Check sheet for the modelled part. Datum: model origin and axes. Units: mm. A direction names the side the tool comes from. Coordinates: 2 decimals unless noted, no trailing zeros. Loops run counter-clockwise (first coordinate to the right, second up) from the corner with the lowest first, then second, coordinate; pieces in that order, holes last.
```python
from build123d import *

# Parameters (mm, degrees)
SKETCH2_R          = 1.5
CUT_EXTRUDE1_DEPTH = 4
SKETCH3_R          = 8.057142585
CUT_EXTRUDE2_DEPTH = 1


with BuildPart() as part:
    # Sketch1 → Revolve2 (revolve)
    with BuildSketch(Plane(origin=(0, 0, 0), x_dir=(0, 0, -1), z_dir=(1, 0, 0))):
        with BuildLine():
            Line((0, 0), (0, 15.5))
            Line((0, 15.5), (2, 15.5))
            Line((2, 15.5), (2, 17.5))
            Line((2, 17.5), (0, 17.5))
            Line((0, 17.5), (0, 20))
            add(Edge.make_bspline(
                [(0, 20), (1.556141404, 22.961218059), (4.442857415, 24.588216471)],
                knots=[0, 0, 0, 1, 1, 1], degree=2))
            Line((4.442857415, 24.588216471), (12.5, 24.588216471))
            Line((12.5, 24.588216471), (12.5, 0))
            Line((12.5, 0), (0, 0))
        make_face()
    revolve(axis=Axis((0, 24.588216471, -12.5), (0, -1, 0)))

    # Sketch2 → Cut-Extrude1 (cut)
    with BuildSketch(Plane.XZ):
        with Locations((0, -12.5)):
            Circle(SKETCH2_R)
    extrude(amount=-CUT_EXTRUDE1_DEPTH, mode=Mode.SUBTRACT)

    # Sketch3 → Cut-Extrude2 (cut)
    with BuildSketch(Plane(origin=(0, 24.588216471, 0), x_dir=(1, 0, 0), z_dir=(0, 1, 0))):
        with Locations((0, 12.5)):
            Circle(SKETCH3_R)
    extrude(amount=-CUT_EXTRUDE2_DEPTH, mode=Mode.SUBTRACT)


solid = part.part
```
1) Mould release check, pull along X, two halves, no side actions. Record for faces 4 (the cylindrical face through (0, 2, -14)), 5 (the flat face through (3, 0, -12)), 6 (the cylindrical face through (-8.45, 7.86, -21.71)): +X half, -X half, draft (parallel to the pull), parting line (faces both ways), or undercut.
Answer sheet:
face 4: undercut
face 5: draft
face 6: parting line
2) Scan lines: line 1 (Z direction, x = 0, y = 3.05); line 2 (Z direction, x = 0, y = 24.15); line 3 (Y direction, x = -10.5, z = -18.25). Record each from-to range of solid material in increasing order.
Answer sheet:
line 1: z = -25 to -14, -11 to 0
line 2: z = -21.27 to -20.56, -4.44 to -3.73
line 3: y = 0 to 15.5, 17.5 to 20.91
3) Depth check by flat-ended pin: pin 1 (1.5 mm diameter, centred on x = -3.5, y = 19.5, fed in from +Z); pin 2 (2 mm diameter, centred on x = 2.5, y = 15.5, fed in from -Z); pin 3 (4 mm diameter, centred on y = 19.5, z = -7, fed in from +X). Enter the tip coordinate at first touch or a pass-through.
Answer sheet:
pin 1: stops at z = -0.31
pin 2: stops at z = -24.91
pin 3: stops at x = 12
4) Set-up check for faces 1 (the cylindrical face through (-1.05, 24.1, -20.49)), 2 (the flat face through (0, 4, -12)), 3 (the flat face through (-7, 15.5, -21)): record each of +Z, -Z, +X, -X, +Y, -Y from which the full face is reachable in a straight line by a thin tool's end or side.
Answer sheet:
face 1: +Y
face 2: -Y
face 3: none
5) Section check A-A on y = 14. Enter the section's corners in (x, z).
Answer sheet:
outline: circle Ø25 at (0, -12.5)
